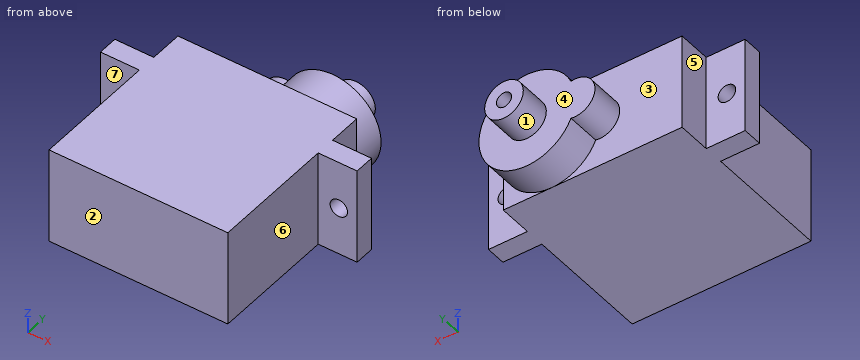
```python
from build123d import *

# Parameters (mm, degrees)
SKETCH2_W           = 22.5
SKETCH2_H           = 12.1
BOSS_EXTRUDE1_DEPTH = 15.7
SKETCH3_W           = 32.3
SKETCH3_H           = 12.1
SKETCH3_R           = 1.1
BOSS_EXTRUDE2_DEPTH = 2.5
SKETCH4_W           = 22.5
SKETCH4_H           = 12.1
BOSS_EXTRUDE3_DEPTH = 4.2
BOSS_EXTRUDE4_DEPTH = 4.3
SKETCH6_R           = 2.43
SKETCH6_R_2         = 0.95
BOSS_EXTRUDE5_DEPTH = 4


with BuildPart() as part:
    # Sketch2 → Boss-Extrude1 (new body)
    with BuildSketch(Plane(origin=(0, 0, 0), x_dir=(1, 0, 0), z_dir=(0, 1, 0))):
        Rectangle(SKETCH2_W, SKETCH2_H)
    extrude(amount=BOSS_EXTRUDE1_DEPTH)

    # Sketch3 → Boss-Extrude2 (add)
    with BuildSketch(Plane(origin=(0, 15.7, 0), x_dir=(1, 0, 0), z_dir=(0, 1, 0))):
        Rectangle(SKETCH3_W, SKETCH3_H)
        with Locations(Location((-13.85, 0, 0), (0, 0, 270))):
            Circle(SKETCH3_R, mode=Mode.SUBTRACT)
        with Locations(Location((13.85, 0, 0), (0, 0, 270))):
            Circle(SKETCH3_R, mode=Mode.SUBTRACT)
    extrude(amount=BOSS_EXTRUDE2_DEPTH)

    # Sketch4 → Boss-Extrude3 (add)
    with BuildSketch(Plane(origin=(0, 18.2, 0), x_dir=(1, 0, 0), z_dir=(0, 1, 0))):
        Rectangle(SKETCH4_W, SKETCH4_H)
    extrude(amount=BOSS_EXTRUDE3_DEPTH)

    # Sketch5 → Boss-Extrude4 (add)
    with BuildSketch(Plane(origin=(0, 22.4, 0), x_dir=(1, 0, 0), z_dir=(0, 1, 0))):
        with BuildLine():
            ThreePointArc((-0.383471074, -2.446057618), (11.2, 0), (-0.383471074, 2.446057618))
            ThreePointArc((-0.383471074, 2.446057618), (-3.4, 0), (-0.383471074, -2.446057618))
        make_face()
    extrude(amount=BOSS_EXTRUDE4_DEPTH)

    # Sketch6 → Boss-Extrude5 (add)
    with BuildSketch(Plane(origin=(0, 26.7, 0), x_dir=(1, 0, 0), z_dir=(0, 1, 0))):
        with Locations(Location((5.15, 0, 0), (0, 0, 270))):
            Circle(SKETCH6_R)
        with Locations(Location((5.15, 0, 0), (0, 0, 270))):
            Circle(SKETCH6_R_2, mode=Mode.SUBTRACT)
    extrude(amount=BOSS_EXTRUDE5_DEPTH)


solid = part.part
```
CAD build for the part. Positions are in the model's coordinates, mm. Face numbers are marked on the shaded views. A direction names the side the tool comes from. Coordinates: 2 decimals unless noted, no trailing zeros. Order: outer loops, then holes, each group sorted by start corner. A loop starts at its lowest first (then second) coordinate and runs counter-clockwise, first axis right, second up. Notation, with made-up numbers: (30, 33.5) -> (88, 33.5) arc R17 cw to (88, 44.5) -> close; hole circle Ø5 at (53.5, -10.5). An arc over 180 degrees is marked (long way). Use one line per item in the form item = value. Start each with the question number.
1) Tool access for the marked faces 4, 5, 6 and 7: list every direction of +Z, -Z, +X, -X, +Y, -Y with a clear straight run to the whole face (end or side of a thin tool).
2) Band-saw the part on B-B on x = 13.85. Give the cut face in (y, z), then the cut area to 4 significant figures.
3) Drill centre lines: L1, parallel to X at y = 16.55, z = 0; L2, parallel to Y at x = -1.5, z = -3.75; L3, parallel to Y at x = 4, z = 2.25. Where is each one in solid material? Low to high. Write a range as [from, to].
4) Band-saw the part on D-D on x = -0.9. Give the cut face in (y, z), then the cut area to 3 significant figures.
5) Band-saw the part on C-C on y = 17. Give the cut face in (x, z).
6) Drop flat-ended pins along their axis: pin 1 (3.5 mm diameter, centred on y = 21.5, z = -3, fed in from +X); pin 2 (5.5 mm diameter, centred on x = 14.5, z = -0.5, fed in from +Y); pin 3 (4 mm diameter, centred on x = -12.5, z = -0.5, fed in from +Y). Give the stop position or say it passes through.
7) Band-saw the part on A-A on z = 0. State how many separate pieces and enclosed holes the cut face has, then the cut area to 3 significant figures.
8) Pull direction Y, two halves, no side cores. Call the marked faces 1, 2 and 3: +Y half, -Y half, draft (parallel to the pull), parting line (faces both ways), or undercut.
Entries:
q1.face_4 = +Y
q1.face_5 = +Z, -Z, -X, +Y
q1.face_6 = +Z, -Z, +X, -Y
q1.face_7 = +Z, -Z, -X, -Y
q2.outline = (15.7, -6.05) -> (18.2, -6.05) -> (18.2, -1.1) -> (15.7, -1.1) -> close; (15.7, 1.1) -> (18.2, 1.1) -> (18.2, 6.05) -> (15.7, 6.05) -> close
q2.area = 24.75 mm2
q3.L1 = [-16.15, -14.95], [-12.75, 12.75], [14.95, 16.15]
q3.L2 = [0, 22.4]
q3.L3 = [0, 26.7]
q4.outline = (0, -6.05) -> (22.4, -6.05) -> (22.4, -2.5) -> (26.7, -2.5) -> (26.7, 2.5) -> (22.4, 2.5) -> (22.4, 6.05) -> (0, 6.05) -> close
q4.area = 293 mm2
q5.outline = (-16.15, -6.05) -> (16.15, -6.05) -> (16.15, 6.05) -> (-16.15, 6.05) -> close; hole circle Ø2.2 at (-13.85, 0); hole circle Ø2.2 at (13.85, 0)
q6.pin_1 = 11.25
q6.pin_2 = 18.2
q6.pin_3 = 22.4
q7.separate_pieces = 3
q7.enclosed_holes = 0
q7.area = 592 mm2
q8.face_1 = draft
q8.face_2 = -Y half
q8.face_3 = +Y half
